from build123d import *

# Parameters (mm, degrees)
SKETCH2_R          = 1.8034
CUT_EXTRUDE1_DEPTH = 5.08
CIRPATTERN2_COUNT  = 4
CHAMFER1_SIZE      = 0.396875


with BuildPart() as part:
    # Sketch1 → Revolve1 (revolve)
    with BuildSketch(Plane.XY):
        with BuildLine():
            Line((-19.670349573, 0), (-19.670349573, 8.580640426))
            Line((-19.670349573, 8.580640426), (-10.272349573, 8.580640426))
            Line((-10.272349573, 8.580640426), (-10.272349573, 11.684))
            Line((-10.272349573, 11.684), (8.777650427, 11.684))
            Line((8.777650427, 11.684), (8.777650427, 14.732))
            Line((8.777650427, 14.732), (43.829650427, 14.732))
            Line((43.829650427, 14.732), (43.829650427, 22.098))
            Line((43.829650427, 22.098), (48.909650427, 22.098))
            Line((48.909650427, 22.098), (48.909650427, 7.055193239))
            add(Edge.make_bspline(
                [(48.909650427, 7.055193239), (50.745745469, 9.469407322), (54.078310122, 11.43), (57.155980429, 11.43)],
                knots=[0, 0, 0, 0, 1, 1, 1, 1], degree=3))
            Line((57.155980429, 11.43), (127.729650427, 11.43))
            ThreePointArc((127.729650427, 11.43), (131.265184333, 9.965533906), (132.729650427, 6.43))
            Line((132.729650427, 6.43), (132.729650427, 0))
            Line((132.729650427, 0), (-19.670349573, 0))
        make_face()
    revolve(axis=Axis((-19.670349573, 0, 0), (1, 0, 0)))

    # Sketch2 → Cut-Extrude1 (cut)
    with BuildSketch(Plane(origin=(48.909650427, 0, 0), x_dir=(0, 0, -1), z_dir=(1, 0, 0))):
        with Locations((0, 19.05)):
            Circle(SKETCH2_R)
    cut_extrude1 = extrude(amount=-CUT_EXTRUDE1_DEPTH, mode=Mode.SUBTRACT)

    # CirPattern2: Cut-Extrude1 ×4 about axis
    cirpattern2_axis = Axis((0, 0, 0), (1, 0, 0))
    for i in range(1, CIRPATTERN2_COUNT):
        add(cut_extrude1.rotate(cirpattern2_axis, i * 360 / CIRPATTERN2_COUNT), mode=Mode.SUBTRACT)

    # Chamfer1
    chamfer1_edges = [part.edges().sort_by_distance(p)[0] for p in [
        (48.909650427, -22.098, 0),
        (43.829650427, -22.098, 0),
        (8.777650427, -14.732, 0),
        (-10.272349573, -11.684, 0),
        (-19.670349573, -8.580640426, 0),
    ]]
    chamfer(chamfer1_edges, length=CHAMFER1_SIZE)


solid = part.part
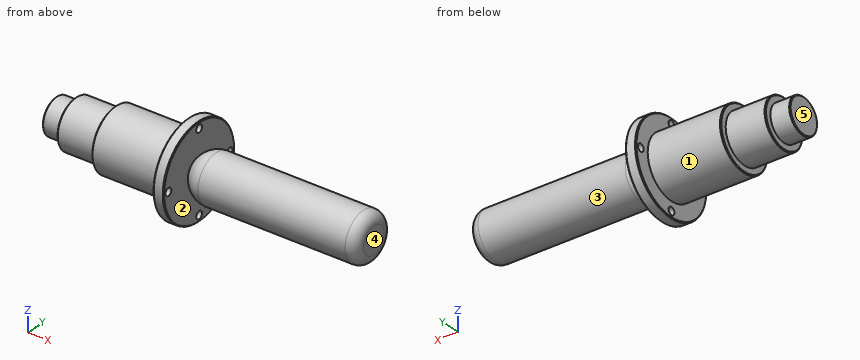
Input: part model. Units: mm. Frame: model coordinates. Face numbers are marked on the shaded views. A direction names the side the tool comes from. Coordinates: 2 decimals unless noted, no trailing zeros. Loops run counter-clockwise (first coordinate to the right, second up) from the corner with the lowest first, then second, coordinate; pieces in that order, holes last.
(1) Section B-B on x = 40.5. Return the cut outline in (y, z).
(2) Section A-A on y = 0. Count the separate pieces of the cut face and the enclosed holes in it, then the cut area to 3 significant figures.
(3) Material intervals for probe 1 along Z at (x, y) = (45.05, 0); probe 2 along Y at (x, z) = (46, 19); probe 3 along X at (y, z) = (17, -7), sorted ascending.
(4) Set-up query: the marked faces 1, 2, 3, 4 and 5. Return all of +Z, -Z, +X, -X, +Y, -Y with unobstructed straight access to the full face (end or side cutting, diameter ignored); none if empty.
(5) First-contact query: pin 1 Ø3 at (y, z) = (-11, -2) entering from -X; pin 2 Ø13 at (y, z) = (-10, 4.5) entering from +X; pin 3 Ø12 at (y, z) = (15, 5) entering from +X; pin 4 Ø4 at (y, z) = (19.05, 0) entering from +X. Flat tips, straight axial feed; report the tip coordinate or a pass-through.
Data:
1. outline: circle Ø29.46 at (0, 0)
2. separate pieces: 3
2. enclosed holes: 0
2. area: 3,710 mm2
3. probe 1: z = -22.1 to -20.85, -17.25 to 17.25, 20.85 to 22.1
3. probe 2: y = -11.28 to -1.8, 1.8 to 11.28
3. probe 3: x = 43.83 to 48.91
4. face 1: -X
4. face 2: none
4. face 3: +X
4. face 4: +Z, -Z, +X, +Y, -Y
4. face 5: +Z, -Z, -X, +Y, -Y
5. pin 1: stops at x = -10.27
5. pin 2: stops at x = 132.73
5. pin 3: stops at x = 131.41
5. pin 4: stops at x = 48.91
